from build123d import *

# Parameters (mm, degrees)
F0_W      = 117.475
F0_H      = 63.5
F1_DEPTH  = 12.7
F2_W      = 57.15
F2_H      = 44.45
F3_DEPTH  = 12.7
F4_W      = 60.325
F4_H      = 44.45
F5_DEPTH  = 34.925
F6_R      = 9.525
F7_DEPTH  = 25.4
F8_R      = 15.875
F9_DEPTH  = 12.7
F10_R     = 9.525
F11_DEPTH = 50.8


with BuildPart() as f1:
    # F0 (on Top) → F1 (new body)
    with BuildSketch(Plane.XY):
        with Locations((58.7375, 31.75)):
            Rectangle(F0_W, F0_H)
    extrude(amount=F1_DEPTH)

    # F2 (on face) → F3 (join)
    with BuildSketch(Plane.XY.offset(12.7)):
        with Locations((28.575, 31.75)):
            Rectangle(F2_W, F2_H)
    extrude(amount=F3_DEPTH)

    # F4 (on face) → F5 (join)
    with BuildSketch(Plane.XY.offset(12.7)):
        with Locations((87.3125, 31.75)):
            Rectangle(F4_W, F4_H)
    extrude(amount=F5_DEPTH)

    # F6 (on face) → F7 (cut)
    with BuildSketch(Plane.XY.offset(25.4)):
        with Locations((31.75, 31.75)):
            Circle(F6_R)
    extrude(amount=-F7_DEPTH, mode=Mode.SUBTRACT)

    # F8 (on face) → F9 (cut)
    with BuildSketch(Plane.XY.offset(47.625)):
        with Locations((87.2998, 31.75)):
            Circle(F8_R)
    extrude(amount=-F9_DEPTH, mode=Mode.SUBTRACT)

    # F10 (on face) → F11 (cut)
    with BuildSketch(Plane.XY.offset(34.925)):
        with Locations((87.2998, 31.75)):
            Circle(F10_R)
    extrude(amount=-F11_DEPTH, mode=Mode.SUBTRACT)


solid = f1.part
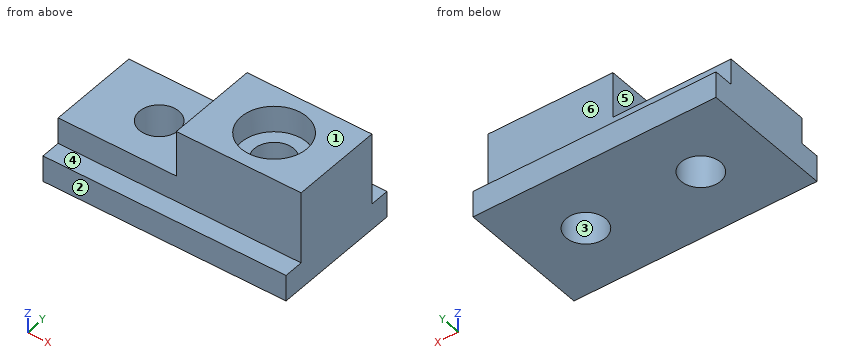
Read the model definition and answer for the solid it produces. Units are mm, in the model's axes. Face numbers are marked on the shaded views. A direction names the side the tool comes from. Coordinates: 2 decimals unless noted, no trailing zeros. Loops run counter-clockwise (first coordinate to the right, second up) from the corner with the lowest first, then second, coordinate; pieces in that order, holes last.
Q1. Consider probe 1 along X at (y, z) = (40, 17) (3 decimals); probe 2 along X at (y, z) = (53, 29) (3 decimals); probe 3 along Y at (x, z) = (31.75, 5.5) (3 decimals). Determine where each line is inside the solid, lowest interval first.
Q2. The part is cut by section D-D on x = 60.5. Write down the section's boundary in (y, z) (3 decimals).
Q3. Each of these flat-tipped pins is pushed along its axis until it touches: pin 1 Ø12 at (x, y) = (40, 27) entering from +Z; pin 2 Ø5 at (x, y) = (83, 5) entering from +Z; pin 3 Ø10.5 at (x, z) = (52.5, 29.5) entering from +Y (3 decimals). Where does it stop, or does it pass through?
Q4. The part is cut by section B-B on y = 31.75. Write down the section's boundary in (x, z) (3 decimals), and give its area (3 significant figures).
Q5. The mould has two halves that part along Y. Classify the marked faces 1, 2 and 3: +Y half, -Y half, draft (parallel to the pull), parting line (faces both ways), or undercut.
Q6. The part is cut by section A-A on x = 31.75. Write down the section's boundary in (y, z) (3 decimals), and give its area (3 significant figures).
Q7. Which of the six approach directions +Z, -Z, +X, -X, +Y, -Y give full straight-line access (tool end or side, diameter ignored) to the marked faces 4, 5 and 6?
Q8. The part is cut by section C-C on z = 28.5. Write down the section's boundary in (x, y) (3 decimals), and give its area (3 significant figures).
Results below:
1. probe 1: x = 0 to 26.989, 36.511 to 82.539, 92.06 to 117.475
1. probe 2: x = 57.15 to 117.475
1. probe 3: y = 0 to 22.225, 41.275 to 63.5
2. outline: (0, 0) - (63.5, 0) - (63.5, 12.7) - (53.975, 12.7) - (53.975, 47.625) - (9.525, 47.625) - (9.525, 12.7) - (0, 12.7) - close
3. pin 1: stops at z = 25.4
3. pin 2: stops at z = 12.7
3. pin 3: stops at y = 53.975
4. outline: (0, 0) - (22.225, 0) - (22.225, 25.4) - (0, 25.4) - close; (41.275, 0) - (77.775, 0) - (77.775, 34.925) - (71.425, 34.925) - (71.425, 47.625) - (57.15, 47.625) - (57.15, 25.4) - (41.275, 25.4) - close; (96.825, 0) - (117.475, 0) - (117.475, 47.625) - (103.175, 47.625) - (103.175, 34.925) - (96.825, 34.925) - close
4. area: 2,770 mm2
5. face 1: draft
5. face 2: -Y half
5. face 3: undercut
6. outline: (0, 0) - (22.225, 0) - (22.225, 25.4) - (9.525, 25.4) - (9.525, 12.7) - (0, 12.7) - close; (41.275, 0) - (63.5, 0) - (63.5, 12.7) - (53.975, 12.7) - (53.975, 25.4) - (41.275, 25.4) - close
6. area: 887 mm2
7. face 4: +Z, +X, -X, -Y
7. face 5: +Z, -X, +Y, -Y
7. face 6: +Z, +X, -X, +Y
8. outline: (57.15, 9.525) - (117.475, 9.525) - (117.475, 53.975) - (57.15, 53.975) - close; hole circle Ø19.05 at (87.3, 31.75)
8. area: 2,400 mm2
